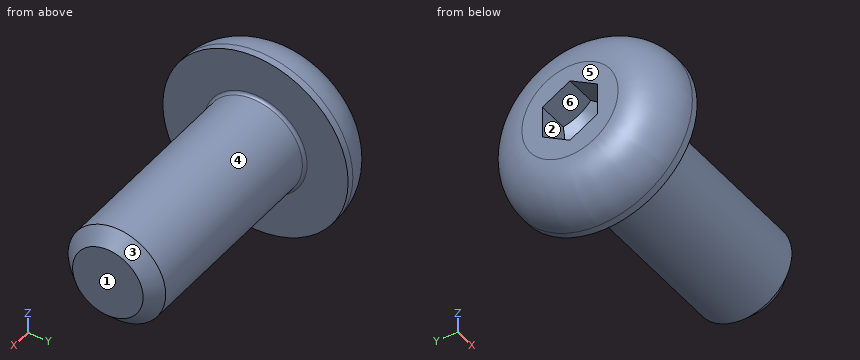
Autodesk Inventor part; units mm, degrees
ref_plane "Work Plane1" through (29, 0, 0) normal (0, -1, 0) x (1, 0, 0)
ref_plane "YZ Plane" through (0, 0, 0) normal (1, 0, 0) x (0, 1, 0)
ref_plane "XZ Plane" through (0, 0, 0) normal (0, 1, 0) x (-1, 0, 0)
sketch "Sketch1" plane through (0, 0, 0) normal (0, 0, 1) x (1, 0, 0)
  line L0 (-0.0762, 0) -> (7.9375, 0)
  line L1 (7.9375, 0) -> (7.9375, 1.7526)
  line L2 (7.9375, 1.7526) -> (1.5902, 1.7526)
  line L3 (1.5902, 1.7526) -> (0.0001, 1.7526)
  line L4 (0.0001, 1.7526) -> (0, 1.7526)
  line L5 (0, 1.7526) -> (0, 3.3274)
  line L6 (0, 3.3274) -> (-1.8542, 3.3274)
  line L7 (-1.8542, 3.3274) -> (-1.8542, 1.1438)
  line L8 (-1.8542, 1.1438) -> (-0.7366, 1.1438)
  line L9 (-0.7366, 1.1438) -> (-0.0762, 0)
  line L10 (-3.8125, 0) -> (9.8958, 0)
  line L11 (0, -0.6655) -> (0, 3.9929)
  line L12 (1.5902, 1.7526) -> (0, 1.7526) construction
  dimension "d1" = 6.3473
  dimension "d2" = 1.5901
  dimension "d3" = 1.8542
  dimension "d4" = 1.1176
  dimension "d5" = 60
  dimension "d6" = 3.5052
  dimension "d7" = 3.5052
  dimension "d8" = 2.2877
  dimension "d9" = 6.6548
  dimension "d26" = 7.9375
revolve "Body" add sketch "Sketch1" angle 360 about axis through (-0.0762, 0, 0) along (1, 0, 0)
sketch "Sketch2" plane through (-1.8542, 0, 0) normal (-1, 0, 0) x (0, 0, 1)
  circle A0 centre (0, 0) radius 1.1438
  line L0 (0, -4.6584) -> (0, 4.6584)
  line L1 (-4.6584, 0) -> (4.6584, 0)
  line L2 (1.1438, 0) -> (0.5719, -0.9906)
  line L3 (0.5719, -0.9906) -> (-0.5719, -0.9906)
  line L4 (-0.5719, -0.9906) -> (-1.1438, 0)
  line L5 (-1.1438, 0) -> (-0.5719, 0.9906)
  line L6 (-0.5719, 0.9906) -> (0.5719, 0.9906)
  line L7 (0.5719, 0.9906) -> (1.1438, 0)
  point P0 (0, 0)
extrude "Slot" add sketch "Sketch2" against normal up to next contours L7 A0 | A0 L2 | L6 L0 A0 | A0 L0 L3 | L0 L6 A0 | A0 L3 L0 | L4 A0 | A0 L5
fillet "Fillet1" radius 1.6002 1 edges at (-1.8542, -3.3274, 0)
thread "Thread"
chamfer "Chamfer1" distance 0.4869 distance2 0.4869 1 edges at (7.9375, -1.7526, 0) measured on face at (7.9375, -0.5672, -0.1398)
ref_plane "Work Plane1" through (29, 0, 0) normal (0, -1, 0) x (1, 0, 0)
fillet "Fillet2" radius 0.1 1 edges at (0.0001, -1.7526, 0)
equation "\"d1\" = GEL"
equation "\"d3\" = KOH"
equation "\"d4\" = INTI"
equation "\"d6\" = GD"
equation "\"d7\" = BDM"
equation "\"d8\" = 1.1547 * SW"
equation "\"d9\" = KOD"
equation "\"d26\" = NLG"
equation "\"d30\" = R"
equation "\"d17\" = RR"
equation "\"d13\" = GEL"
equation "\"d15\" = -0.5 * SPD + 0.5 * GD"
equation "\"d16\" = GUL"
equation "\"GD\" = NND"
equation "\"NLG\" = 7.9375"
equation "\"GEL\" = 6.34726"
equation "\"KOD\" = 6.6548"
equation "\"KOH\" = 1.8542"
equation "\"INTI\" = 1.1176"
equation "\"GAL\" = 1.59004"
equation "\"GUL\" = 0.48692"
equation "\"BDM\" = NND"
equation "\"SW\" = 1.9812"
equation "\"RR\" = 1.6002"
equation "\"SPD\" = 2.53136"
equation "\"R\" = 0.1"
equation "\"TOA\" = 30deg"
equation "\"GD1\" = SPD"
equation "\"THREADDIA\" = 3.5052"
equation "\"KOH1\" = 0.381"
equation "\"NND\" = 3.5052"
equation "\"E0\" = 2.28829"
properties part number "ANSI B18.3 - 6 - 32 x 5/16" material "Steel, Mild"
Read the model definition and answer for the solid it produces. Units are mm, in the model's axes. Face numbers are marked on the shaded views. A direction names the side the tool comes from. Give positions to 0.01 mm unless a question says otherwise; leave off trailing zeros. Write each loop counter-clockwise with the first axis right and the second up, starting at its lowest first coordinate (ties: lowest second). Pieces come first, ordered by that corner, then holes. Notation, with made-up numbers: M 11.25,10 L 36.25,10 A21 ccw 36.25,46 Z; hole C -35.75,50.25 d11. An arc over 180 degrees is marked long. One line per item, written item: value. Start each with the question number.
(1) A tool of negligible diameter and unlimited length cuts with its end or side. For the marked faces 4, 5 and 6, from which of +Z, -Z, +X, -X, +Y, -Y can it reach the whole face along a straight path? Write none if from no direction.
(2) Find the intervals of material crossed by line 1 (Y direction, x = 0.75, z = 0); line 2 (Z direction, x = -0.5, y = -1.75), in increasing order.
(3) Flat-ended cylindrical pins translate along their axes: pin 1 Ø1.3 at (x, z) = (-1.5, 0) entering from +Y; pin 2 Ø1.5 at (y, z) = (2, -2.5) entering from -X. Find the tip coordinate at first contact, or state that the pin passes through.
(4) Find section A-A (x = 4.5). Determine the outline of the cut face in (y, z), plus the area to 3 significant figures.
(5) Determine the mould class of the marked faces 1, 2 and 3 for opening direction Z: pulls with the +Z half, pulls with the -Z half, needs draft (parallel to the pull), parting line crosses it, or undercut.
Results below:
1. face 4: +X
1. face 5: +Z, -Z, -X, +Y, -Y
1. face 6: -X
2. line 1: y = -1.75 to 1.75
2. line 2: z = -2.81 to 2.81
3. pin 1: stops at y = 3.21
3. pin 2: stops at x = -1.68
4. outline: C 0,0 d3.51
4. area: 9.65 mm^2
5. face 1: needs draft
5. face 2: undercut
5. face 3: parting line crosses it
